The listing builds one solid part. Answer for the finished solid, in the listing's coordinates (mm). Face numbers are marked on the shaded views. A direction names the side the tool comes from. Give positions to 0.01 mm unless a question says otherwise; leave off trailing zeros. Write each loop counter-clockwise with the first axis right and the second up, starting at its lowest first coordinate (ties: lowest second). Pieces come first, ordered by that corner, then holes. Notation, with made-up numbers: (51, -31.75) -> (82, -31.75) arc R17 ccw to (82, -25.75) -> close; hole circle Ø2 at (80, -30.75). An arc over 180 degrees is marked (long way). Write each question's results on one line, items separated by ' | '. Start each with the question number.
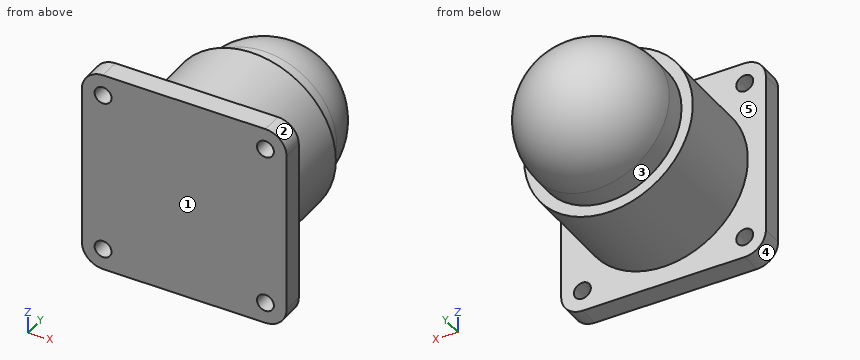
from build123d import *

# Parameters (mm, degrees)
SKETCH1_W           = 29
SKETCH1_H           = 29
SKETCH1_R           = 1.2
BOSS_EXTRUDE1_DEPTH = 3
FILLET1_R           = 3
SKETCH2_R           = 11.95
BOSS_EXTRUDE2_DEPTH = 13.5
SKETCH3_R           = 10.35
BOSS_EXTRUDE3_DEPTH = 3


with BuildPart() as part:
    # Sketch1 → Boss-Extrude1 (new body)
    with BuildSketch(Plane(origin=(0, 0, 0), x_dir=(1, 0, 0), z_dir=(0, 1, 0))):
        with Locations((14.5, 14.5)):
            Rectangle(SKETCH1_W, SKETCH1_H)
        with Locations((3, 26)):
            Circle(SKETCH1_R, mode=Mode.SUBTRACT)
        with Locations((26, 26)):
            Circle(SKETCH1_R, mode=Mode.SUBTRACT)
        with Locations((26, 3)):
            Circle(SKETCH1_R, mode=Mode.SUBTRACT)
        with Locations((3, 3)):
            Circle(SKETCH1_R, mode=Mode.SUBTRACT)
    extrude(amount=BOSS_EXTRUDE1_DEPTH)

    # Fillet1
    fillet1_edges = [part.edges().sort_by_distance(p)[0] for p in [
        (0, 1.5, -29),
        (29, 1.5, -29),
        (29, 1.5, 0),
        (0, 1.5, 0),
    ]]
    fillet(fillet1_edges, radius=FILLET1_R)

    # Sketch2 → Boss-Extrude2 (add)
    with BuildSketch(Plane(origin=(0, 3, 0), x_dir=(1, 0, 0), z_dir=(0, 1, 0))):
        with Locations((14.5, 14.5)):
            Circle(SKETCH2_R)
    extrude(amount=BOSS_EXTRUDE2_DEPTH)

    # Sketch3 → Boss-Extrude3 (add)
    with BuildSketch(Plane(origin=(0, 16.5, 0), x_dir=(1, 0, 0), z_dir=(0, 1, 0))):
        with Locations((14.5, 14.5)):
            Circle(SKETCH3_R)
    extrude(amount=BOSS_EXTRUDE3_DEPTH)

    # Sketch4 → Revolve1 (revolve)
    with BuildSketch(Plane.XY.offset(-14.5)):
        with BuildLine():
            Line((14.5, 19.5), (14.5, 29.85))
            ThreePointArc((14.5, 29.85), (21.818555185, 26.818555185), (24.85, 19.5))
            Line((24.85, 19.5), (14.5, 19.5))
        make_face()
    revolve(axis=Axis((14.5, 19.5, -14.5), (0, 1, 0)))


solid = part.part
1. Section C-C (y = 23.75) is taken. Write down the section's boundary in (x, z), then the cut area to 3 significant figures.
2. A tool of negligible diameter and unlimited length cuts with its end or side. For the marked faces 4 and 5, from which of +Z, -Z, +X, -X, +Y, -Y can it reach the whole face along a straight path? Write none if from no direction.
3. Consider probe 1 along Z at (x, y) = (3, 0.95); probe 2 along X at (y, z) = (1, -26); probe 3 along Y at (x, z) = (25, -7.25). Determine where each line is inside the solid, lowest interval first. Write a range as [from, to].
4. Section B-B (x = 14.5) is taken. Write down the section's boundary in (y, z), then the cut area to 3 significant figures.
5. The mould has two halves that part along X. Classify the marked faces 1, 2 and 3: pulls with the +X half, pulls with the -X half, needs draft (parallel to the pull), parting line crosses it, or undercut.
6. Section A-A (z = -14.5) is taken. Write down the section's boundary in (x, y).
7. Each of these flat-tipped pins is pushed along its axis until it touches: pin 1 Ø8 at (y, z) = (14, -23.5) entering from +X; pin 2 Ø2 at (x, z) = (23.5, -14) entering from +Y; pin 3 Ø12 at (y, z) = (15.5, -22) entering from -X; pin 4 Ø1.9 at (x, z) = (26, -26) entering from +Y. Where does it stop, or does it pass through?
Results:
1) outline: circle Ø18.87 at (14.5, -14.5) | area: 280 mm²
2) face 4: -Z, -X, +Y, -Y | face 5: +Y
3) probe 1: z = [-29, -27.2], [-24.8, -4.2], [-1.8, 0] | probe 2: x = [0, 1.8], [4.2, 24.8], [27.2, 29] | probe 3: y = [0, 3]
4) outline: (0, -29) -> (3, -29) -> (3, -26.45) -> (16.5, -26.45) -> (16.5, -24.85) -> (19.5, -24.85) arc R10.35 ccw to (19.5, -4.15) -> (16.5, -4.15) -> (16.5, -2.55) -> (3, -2.55) -> (3, 0) -> (0, 0) -> close | area: 640 mm²
5) face 1: needs draft | face 2: pulls with the +X half | face 3: parting line crosses it
6) outline: (0, 0) -> (29, 0) -> (29, 3) -> (26.45, 3) -> (26.45, 16.5) -> (24.85, 16.5) -> (24.85, 19.5) arc R10.35 ccw to (4.15, 19.5) -> (4.15, 16.5) -> (2.55, 16.5) -> (2.55, 3) -> (0, 3) -> close
7) pin 1: stops at x = 25.35 | pin 2: stops at y = 26.05 | pin 3: stops at x = 2.64 | pin 4: passes through
